Could you check a few things on this model? Use its own coordinates, in mm. A direction names the side the tool comes from. Coordinates: 2 decimals unless noted, no trailing zeros. Order: outer loops, then holes, each group sorted by start corner. A loop starts at its lowest first (then second) coordinate and runs counter-clockwise, first axis right, second up. Notation, with made-up numbers: (-25, 8) -> (23, 8) arc R33 ccw to (23, 47) -> close; hole circle Ø11 at (-5.75, 30.5). An arc over 180 degrees is marked (long way). Return JSON: item names as keys, results as strings. Group by question number.
from build123d import *

# Parameters (mm, degrees)
BOSS_EXTRUDE1_DEPTH = 18
CUT_EXTRUDE1_DEPTH  = 18
CUT_EXTRUDE2_DEPTH  = 18
SKETCH4_W           = 45.12531779
SKETCH4_H           = 70
CUT_EXTRUDE3_DEPTH  = 7
SKETCH5_R           = 2.5
CUT_EXTRUDE4_DEPTH  = 70
SKETCH6_W           = 143.844268465
SKETCH6_H           = 20
CUT_EXTRUDE5_DEPTH  = 15


with BuildPart() as part:
    # Sketch1 → Boss-Extrude1 (new body)
    with BuildSketch(Plane(origin=(0, 0, 0), x_dir=(1, 0, 0), z_dir=(0, 1, 0))):
        with BuildLine():
            Line((-90.5, -20), (-90.5, 20))
            ThreePointArc((-90.5, 20), (-86.106601718, 30.606601718), (-75.5, 35))
            Line((-75.5, 35), (75.5, 35))
            ThreePointArc((75.5, 35), (86.106601718, 30.606601718), (90.5, 20))
            Line((90.5, 20), (90.5, -20))
            ThreePointArc((90.5, -20), (86.106601718, -30.606601718), (75.5, -35))
            Line((75.5, -35), (-75.5, -35))
            ThreePointArc((-75.5, -35), (-86.106601718, -30.606601718), (-90.5, -20))
        make_face()
    extrude(amount=BOSS_EXTRUDE1_DEPTH)

    # Sketch3 → Cut-Extrude1 (cut)
    with BuildSketch(Plane(origin=(0, 18, 0), x_dir=(1, 0, 0), z_dir=(0, 1, 0))):
        Polygon((-75.5, 35), (-68.344268465, 20), (-53.344268465, 35), align=None)
    extrude(amount=-CUT_EXTRUDE1_DEPTH, mode=Mode.SUBTRACT)

    # Sketch3<3> → Cut-Extrude2 (cut)
    with BuildSketch(Plane(origin=(0, 18, 0), x_dir=(1, 0, 0), z_dir=(0, 1, 0))):
        Polygon((-75.5, 35), (-68.344268465, 20), (-53.344268465, 35), align=None)
        Polygon((-75.5, -35), (-68.344268465, -20), (-53.344268465, -35), align=None)
    extrude(amount=-CUT_EXTRUDE2_DEPTH, mode=Mode.SUBTRACT)

    # Sketch4 → Cut-Extrude3 (cut)
    with BuildSketch(Plane(origin=(0, 18, 0), x_dir=(1, 0, 0), z_dir=(0, 1, 0))):
        with Locations((-75.90692736, 0)):
            Rectangle(SKETCH4_W, SKETCH4_H)
    extrude(amount=-CUT_EXTRUDE3_DEPTH, mode=Mode.SUBTRACT)

    # Sketch5 → Cut-Extrude4 (cut)
    with BuildSketch(Plane.XY.offset(35)):
        with Locations((-75.5, 5.5)):
            Circle(SKETCH5_R)
    extrude(amount=-CUT_EXTRUDE4_DEPTH, mode=Mode.SUBTRACT)

    # Sketch6 → Cut-Extrude5 (cut)
    with BuildSketch(Plane(origin=(0, 18, 0), x_dir=(1, 0, 0), z_dir=(0, 1, 0))):
        with Locations((18.577865767, 0)):
            Rectangle(SKETCH6_W, SKETCH6_H)
    extrude(amount=-CUT_EXTRUDE5_DEPTH, mode=Mode.SUBTRACT)


solid = part.part
Q1. I want a section at A-A on y = 13.5. Please give me the cut outline in (x, z).
Q2. I want a section at B-B on z = 2.5. Please give me the cut outline in (x, y).
Q3. We'd pull the mould along Z, two halves only. Please class faces 1 (the cylindrical face through (-86.22, 5.42, -30.49)), 2 (the cylindrical face through (86.22, 8.87, 30.49)), 3 (the flat face through (-53.344, 15, 23)), 4 (the flat face through (-53.344, 7, 0)): pulls with the +Z half, pulls with the -Z half, needs draft (parallel to the pull), parting line crosses it, or undercut.
Q4. I want a section at D-D on y = 5.5. Please give me the cut outline in (x, z), and give its area (3 significant figures).
Q5. On a 3-axis mill with a long thin cutter (end or side, diameter ignored), from which of +Z, -Z, +X, -X, +Y, -Y can I reach the whole of each face in a straight line? I mean faces 5 (the flat face through (18, 11, -10)), 6 (the flat face through (-71.97, 5.58, 27.6)), 7 (the flat face through (-72, 11, 0)). Say none if no direction works.
Q6. I need wall thicknesses on line 1 along Z through (x, y) = (72.5, 6.5); line 2 along Y through (x, z) = (-75.5, 0); line 3 along X through (y, z) = (5.5, -5). Which ranges of each line are inside material? Lowest first, please. Write a range as from..to.
Q7. I want a section at C-C on x = 16. Please give me the cut outline in (y, z).
Q8. I'm going to push flat-ended pins straight in: pin 1 Ø12 at (x, z) = (-65, 15) entering from +Y; pin 2 Ø5.5 at (y, z) = (16, -22) entering from -X; pin 3 Ø10 at (x, z) = (12, 4.5) entering from +Y. Where does each tip first touch, or does it pass through?
Response values:
{
 "1": {"outline": "(-53.34, -35) -> (75.5, -35) arc R15 ccw to (90.5, -20) -> (90.5, -10) -> (-53.34, -10) -> close; (-53.34, 10) -> (90.5, 10) -> (90.5, 20) arc R15 ccw to (75.5, 35) -> (-53.34, 35) -> close"},
 "2": {"outline": "(-90.5, 0) -> (90.5, 0) -> (90.5, 3) -> (-53.34, 3) -> (-53.34, 11) -> (-90.5, 11) -> close; hole circle Ø5 at (-75.5, 5.5)"},
 "3": {"face 1": "pulls with the -Z half", "face 2": "pulls with the +Z half", "face 3": "needs draft", "face 4": "undercut"},
 "4": {"outline": "(-90.5, -20) arc R15 ccw to (-78, -34.79) -> (-78, 34.79) arc R15 ccw to (-90.5, 20) -> close; (-73, -29.76) -> (-68.34, -20) -> (-53.34, -35) -> (75.5, -35) arc R15 ccw to (90.5, -20) -> (90.5, -10) -> (-53.34, -10) -> (-53.34, 10) -> (90.5, 10) -> (90.5, 20) arc R15 ccw to (75.5, 35) -> (-53.34, 35) -> (-68.34, 20) -> (-73, 29.76) -> close", "area": "8,930 mm²"},
 "5": {"face 5": "+X, +Y", "face 6": "+Z, +Y, -Y", "face 7": "+Z, -Z, -X, +Y"},
 "6": {"line 1": "z = -35..-10, 10..35", "line 2": "y = 0..3, 8..11", "line 3": "x = -90.5..-78, -73..-53.34"},
 "7": {"outline": "(0, -35) -> (18, -35) -> (18, -10) -> (3, -10) -> (3, 10) -> (18, 10) -> (18, 35) -> (0, 35) -> close"},
 "8": {"pin 1": "stops at y = 11", "pin 2": "stops at x = -53.34", "pin 3": "stops at y = 3"}
}
